```python
from build123d import *

# Parameters (mm, degrees)
F0_W     = 79.8
F0_H     = 79.8
F1_DEPTH = 48
F2_W     = 74
F2_H     = 74
F3_DEPTH = 45
F4_R     = 4
F5_R     = 1
F6_T     = -1


with BuildPart() as f1:
    # F0 (on Top) → F1 (new body)
    with BuildSketch(Plane.XY):
        Rectangle(F0_W, F0_H)
    extrude(amount=F1_DEPTH)

    # F2 (on face) → F3 (cut)
    with BuildSketch(Plane.XY.offset(48)):
        Rectangle(F2_W, F2_H)
    extrude(amount=-F3_DEPTH, mode=Mode.SUBTRACT)

    # F4
    f4_edges = [f1.edges().sort_by_distance(p)[0] for p in [
        (-39.9, -39.9, 24),
        (39.9, -39.9, 24),
        (39.9, 39.9, 24),
        (-39.9, 39.9, 24),
    ]]
    fillet(f4_edges, radius=F4_R)

    # F5
    f5_edges = [f1.edges().sort_by_distance(p)[0] for p in [
        (-37, -37, 25.5),
        (-37, 37, 25.5),
        (37, 37, 25.5),
        (37, -37, 25.5),
    ]]
    fillet(f5_edges, radius=F5_R)

    # F6
    f6_openings = [f1.faces().sort_by_distance(p)[0] for p in [
        (0, 0, 0),
    ]]
    offset(amount=F6_T, openings=f6_openings, kind=Kind.INTERSECTION)


solid = f1.part
```
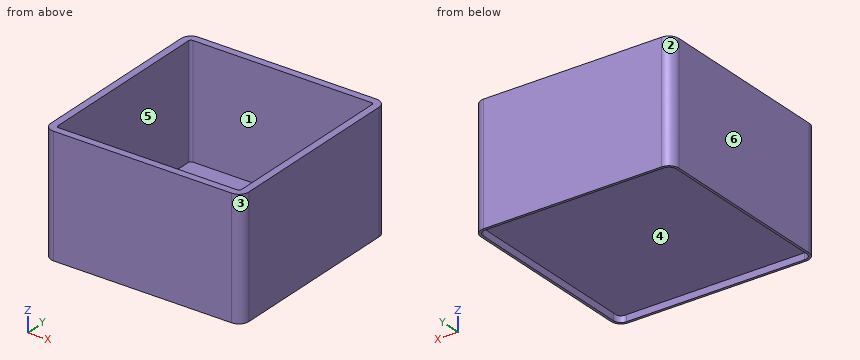
Read the model definition and answer for the solid it produces. Units are mm, in the model's axes. Face numbers are marked on the shaded views. A direction names the side the tool comes from. Give positions to 0.01 mm unless a question says otherwise; leave off trailing zeros. Loops run counter-clockwise (first coordinate to the right, second up) from the corner with the lowest first, then second, coordinate; pieces in that order, holes last.
Item 1: The mould has two halves that part along X. Classify the marked faces 1, 2 and 3: released by +X, released by -X, zero draft, split by the parting line, or undercut.
Item 2: For the marked faces 4, 5 and 6, determine the directions among +Z, -Z, +X, -X, +Y, -Y from which every point of the face is accessible in a straight line to the end or side of a thin tool.
Item 3: Each of these flat-tipped pins is pushed along its axis until it touches: pin 1 Ø1 at (x, y) = (-16, -25) entering from -Z; pin 2 Ø8 at (x, y) = (-21, -12.5) entering from +Z. Where does it stop, or does it pass through?
Item 4: Find the intervals of material crossed by line 1 along X through (y, z) = (-20, 19); line 2 along Z through (x, y) = (33, -25.5), in increasing order.
Item 5: The part is cut by section B-B (y = -21). Write down the section's boundary in (x, z).
Item 6: The part is cut by section A-A (z = 18). Give the number of separate pieces and of enclosed holes in the cut face, and give its area (3 significant figures).
Taken from the geometry:
1. face 1: undercut
1. face 2: released by -X
1. face 3: released by +X
2. face 4: -Z
2. face 5: +Z
2. face 6: +Z, -Z, -X, +Y, -Y
3. pin 1: stops at z = 2
3. pin 2: stops at z = 3
4. line 1: x = -39.9 to -38.9, -38 to -37, 37 to 38, 38.9 to 39.9
4. line 2: z = 2 to 3
5. outline: (-39.9, 0) - (-38.9, 0) - (-38.9, 47) - (-38, 47) - (-38, 2) - (38, 2) - (38, 47) - (38.9, 47) - (38.9, 0) - (39.9, 0) - (39.9, 48) - (37, 48) - (37, 3) - (-37, 3) - (-37, 48) - (-39.9, 48) - close
6. separate pieces: 2
6. enclosed holes: 2
6. area: 607 mm2
